```python
from build123d import *

# Parameters (mm, degrees)
F0_W          = 250
F0_H          = 250
F0_R          = 120
F1_DEPTH      = 20
F0_R_2        = 110
F2_DEPTH      = 15
F2_DEPTH_BACK = 5


with BuildPart() as f1:
    # F0 (on Top) → F1 (new body)
    with BuildSketch(Plane.XY):
        Rectangle(F0_W, F0_H)
        Circle(F0_R, mode=Mode.SUBTRACT)
    extrude(amount=F1_DEPTH)

    # F0 (on Top) → F2 (join, two sides)
    with BuildSketch(Plane.XY) as f2_sk:
        Circle(F0_R)
        Circle(F0_R_2, mode=Mode.SUBTRACT)
    extrude(amount=F2_DEPTH)
    extrude(f2_sk.sketch, amount=-F2_DEPTH_BACK)


solid = f1.part
```
For this review, take the finished solid that the model builds, in its own axes (mm). A direction names the side the tool comes from. Round coordinates to 2 decimals unless told otherwise and drop trailing zeros. Write each loop counter-clockwise with the first axis right and the second up, starting at its lowest first coordinate (ties: lowest second). Pieces come first, ordered by that corner, then holes. Notation, with made-up numbers: (-7.75, -13) - (30.25, -13) arc R30 cw to (30.25, 12) - close; hole circle Ø7 at (29, 88.25). An arc over 180 degrees is marked (long way). Answer as CSV lines item,"result". Start each with the question number.
(1) Machinability: for faces 5 (the flat face through (53, -97, 15)), 6 (the flat face through (-47, -111, 0)), 7 (the flat face through (-2, 125, 10)), which of the approach directions +Z, -Z, +X, -X, +Y, -Y give a long, thin tool a straight path to every point of the face, cutting with its end or side? Answer none if there is none.
(2) Add section A-A, the plane y = 0. State the section outline as (x, z) points.
(3) Mouldability with a two-part tool opening along Y and no side actions: class faces 1 (the cylindrical face through (-119.884, 5.276, -2.465)), 2 (the flat face through (125, -2, 10)), 3 (the cylindrical face through (-119.884, 5.276, 17.465)), 4 (the flat face through (-2, -125, 10)) as +Y half, -Y half, draft (parallel to the pull), parting line (faces both ways), or undercut.
(4) For line 1 (Y direction, x = 0, z = 6.5); line 2 (Y direction, x = 0, z = -3); line 3 (Z direction, x = -42.5, y = 110.5), list the stretches that pass through material, from the lowest coordinate up.
(5) Add section C-C, the plane z = 10.5. State the section outline as (x, y) points, plus the area to 3 significant figures.
From the geometry:
1,face 5,"+Z"
1,face 6,"-Z"
1,face 7,"+Z, -Z, +X, -X, +Y"
2,outline,"(-125, 0) - (-120, 0) - (-120, -5) - (-110, -5) - (-110, 15) - (-120, 15) - (-120, 20) - (-125, 20) - close; (110, -5) - (120, -5) - (120, 0) - (125, 0) - (125, 20) - (120, 20) - (120, 15) - (110, 15) - close"
3,face 1,"parting line"
3,face 2,"draft"
3,face 3,"undercut"
3,face 4,"-Y half"
4,line 1,"y = -125 to -110, 110 to 125"
4,line 2,"y = -120 to -110, 110 to 120"
4,line 3,"z = -5 to 15"
5,outline,"(-125, -125) - (125, -125) - (125, 125) - (-125, 125) - close; hole circle Ø220 at (0, 0)"
5,area,"24,500 mm²"
